Input: part model. Units: mm. Frame: model coordinates. Face numbers are marked on the shaded views. Coordinates: 2 decimals unless noted, no trailing zeros. Loops run counter-clockwise (first coordinate to the right, second up) from the corner with the lowest first, then second, coordinate; pieces in that order, holes last. Notation, with made-up numbers: (-39.75, 79.5) - (5.25, 79.5) arc R19 cw to (5.25, 114.5) - close; hole circle Ø1 at (63.5, 59). An arc over 180 degrees is marked (long way). Use a Markdown table: item, result. Add a question column.
1. Draft query along X for the marked faces 1 and 2. Return one class per face: released by +X, released by -X, zero draft, split by the parting line, or undercut.
2. Section query A-A on y = 30. Return the cut outline in (x, z).
3. Contact query for flat-ended pins moving along their axis: P1, Ø5, axis at x = 8, z = 34.5, coming from the -Y side; P2, Ø10, axis at x = -17, z = 42, coming from the -Y side; P3, Ø1, axis at x = 7.5, z = 27.5, coming from the +Y side. Output: stop coordinate, or through.
4. Ray query, L1, parallel to X at y = -8, z = 49; L2, parallel to X at y = 4.5, z = 46; L3, parallel to Y at x = 7, z = 8.5. Return the intervals inside material, ascending. Write a range as [from, to].
5. Section query B-B on x = 1.5. Return the cut outline in (y, z).
```python
from build123d import *

# Parameters (mm, degrees)
F0_R     = 36.5
F1_DEPTH = 55
F2_R     = 2
F3_R     = 2
F4_R     = 1
F5_R     = 2
F6_R     = 2
F7_R     = 1
F8_R     = 1
F9_R     = 2
F10_R    = 2


with BuildPart() as f1:
    # F0 (on Top) → F1 (new body)
    with BuildSketch(Plane.XY):
        with BuildLine():
            ThreePointArc((31.826434, -18.375), (35.497774, -9.5116), (36.75, 0))
            ThreePointArc((36.75, 0), (27.38989, 24.502172), (4.077541, 36.523091))
            ThreePointArc((4.077541, 36.523091), (2.041925, 36.693229), (0, 36.75))
            ThreePointArc((0, 36.75), (-30.756306, 20.114973), (-33.668695, -14.730292))
            ThreePointArc((-33.668695, -14.730292), (-32.798231, -16.578256), (-31.826434, -18.375))
            ThreePointArc((-31.826434, -18.375), (-2.041925, -36.693229), (29.591154, -21.792799))
            ThreePointArc((29.591154, -21.792799), (30.756306, -20.114973), (31.826434, -18.375))
        make_face()
        Circle(F0_R, mode=Mode.SUBTRACT)
        with BuildLine():
            ThreePointArc((0, 36.75), (2.041925, 36.693229), (4.077541, 36.523091))
            Line((4.077541, 36.523091), (4.077541, 39.312689))
            Line((4.077541, 39.312689), (0, 40.75))
            Line((0, 40.75), (0, 36.75))
        make_face()
        with BuildLine():
            ThreePointArc((-31.826434, -18.375), (-32.798231, -16.578256), (-33.668695, -14.730292))
            Line((-33.668695, -14.730292), (-36.084558, -16.125091))
            Line((-36.084558, -16.125091), (-35.290535, -20.375))
            Line((-35.290535, -20.375), (-31.826434, -18.375))
        make_face()
        with BuildLine():
            Line((35.290535, -20.375), (31.826434, -18.375))
            ThreePointArc((31.826434, -18.375), (30.756306, -20.114973), (29.591154, -21.792799))
            Line((29.591154, -21.792799), (32.007017, -23.187598))
            Line((32.007017, -23.187598), (35.290535, -20.375))
        make_face()
    extrude(amount=F1_DEPTH)

    # F2
    f2_edges = [f1.edges().sort_by_distance(p)[0] for p in [
        (4.077541, 39.312689, 27.5),
    ]]
    fillet(f2_edges, radius=F2_R)

    # F3
    f3_edges = [f1.edges().sort_by_distance(p)[0] for p in [
        (4.077541, 36.523091, 27.5),
    ]]
    fillet(f3_edges, radius=F3_R)

    # F4
    f4_edges = [f1.edges().sort_by_distance(p)[0] for p in [
        (0, 36.75, 27.5),
    ]]
    fillet(f4_edges, radius=F4_R)

    # F5
    f5_edges = [f1.edges().sort_by_distance(p)[0] for p in [
        (32.007017, -23.187598, 27.5),
    ]]
    fillet(f5_edges, radius=F5_R)

    # F6
    f6_edges = [f1.edges().sort_by_distance(p)[0] for p in [
        (29.591154, -21.792799, 27.5),
    ]]
    fillet(f6_edges, radius=F6_R)

    # F7
    f7_edges = [f1.edges().sort_by_distance(p)[0] for p in [
        (31.826434, -18.375, 27.5),
    ]]
    fillet(f7_edges, radius=F7_R)

    # F8
    f8_edges = [f1.edges().sort_by_distance(p)[0] for p in [
        (-31.826434, -18.375, 27.5),
    ]]
    fillet(f8_edges, radius=F8_R)

    # F9
    f9_edges = [f1.edges().sort_by_distance(p)[0] for p in [
        (-36.084558, -16.125091, 27.5),
    ]]
    fillet(f9_edges, radius=F9_R)

    # F10
    f10_edges = [f1.edges().sort_by_distance(p)[0] for p in [
        (-33.668695, -14.730292, 27.5),
    ]]
    fillet(f10_edges, radius=F10_R)


solid = f1.part
```
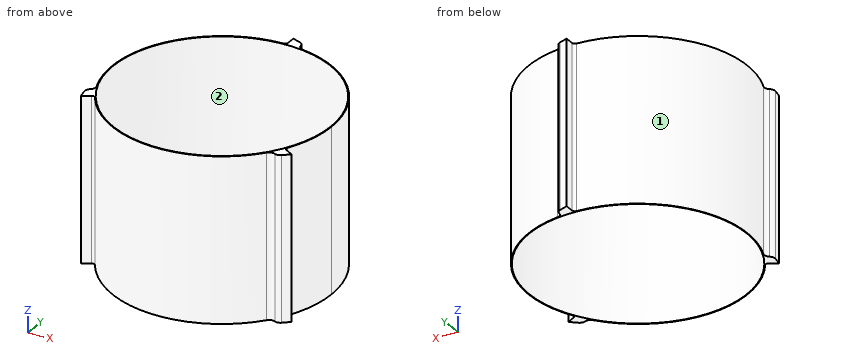
Resolved:
| question | item | result |
|---|---|---|
| 1 | face 1 | released by -X |
| 1 | face 2 | undercut |
| 2 | outline | (-21.23, 0) - (-20.79, 0) - (-20.79, 55) - (-21.23, 55) - close; (20.79, 0) - (21.23, 0) - (21.23, 55) - (20.79, 55) - close |
| 3 | P1 | y = -36.34 |
| 3 | P2 | y = -34.74 |
| 3 | P3 | y = 36.08 |
| 4 | L1 | [-35.87, -35.61], [35.61, 35.87] |
| 4 | L2 | [-36.47, -36.22], [36.22, 36.47] |
| 4 | L3 | [-36.08, -35.82], [35.82, 36.08] |
| 5 | outline | (-36.72, 0) - (-36.47, 0) - (-36.47, 55) - (-36.72, 55) - close; (36.47, 0) - (40.22, 0) - (40.22, 55) - (36.47, 55) - close |
